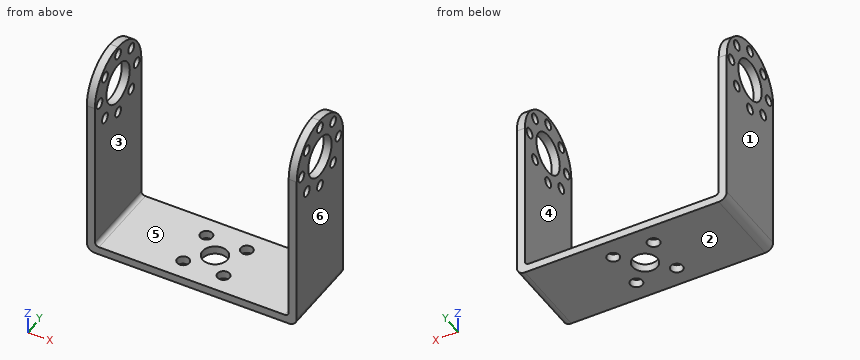
```python
from build123d import *

# Parameters (mm, degrees)
EXTRUDE_1_DEPTH     = 20
FILLET_1_R          = 2
FILLET_2_R          = 1
CUT_EXTRUDE_1_DEPTH = 52
CUT_EXTRUDE_2_DEPTH = 52
SKETCH_4_R          = 5.025
SKETCH_4_R_2        = 1.25
CUT_EXTRUDE_3_DEPTH = 52
CUT_EXTRUDE_4_REACH = 52
SKETCH_5_R          = 3.05
SKETCH_5_R_2        = 1.5


with BuildPart() as part:
    # 草图1 → 凸台-拉伸1 (new body)
    with BuildSketch(Plane(origin=(0, 0, 0), x_dir=(1, 0, 0), z_dir=(0, 1, 0))):
        Polygon((-19.308800698, 32.095662915), (32.691199302, 32.095662915), (32.691199302, -17.904337085), (30.691199302, -17.904337085), (30.691199302, 30.095662915), (-17.308800698, 30.095662915), (-17.308800698, -17.904337085), (-19.308800698, -17.904337085), align=None)
    extrude(amount=EXTRUDE_1_DEPTH)

    # 圆角1
    fillet_1_edges = [part.edges().sort_by_distance(p)[0] for p in [
        (-19.308800698, 10, -32.095662915),
        (32.691199302, 10, -32.095662915),
    ]]
    fillet(fillet_1_edges, radius=FILLET_1_R)

    # 圆角2
    fillet_2_edges = [part.edges().sort_by_distance(p)[0] for p in [
        (30.691199302, 10, -30.095662915),
        (-17.308800698, 10, -30.095662915),
    ]]
    fillet(fillet_2_edges, radius=FILLET_2_R)

    # 草图2 → 切除-拉伸1 (cut)
    with BuildSketch(Plane.ZY.offset(19.308800698)):
        with BuildLine():
            Line((7.904337085, 20), (17.904337085, 20))
            Line((17.904337085, 20), (17.904337085, 10))
            ThreePointArc((17.904337085, 10), (14.975404897, 17.071067812), (7.904337085, 20))
        make_face()
    extrude(amount=-CUT_EXTRUDE_1_DEPTH, mode=Mode.SUBTRACT)

    # 草图3 → 切除-拉伸2 (cut)
    with BuildSketch(Plane.ZY.offset(19.308800698)):
        with BuildLine():
            Line((7.904337085, 0), (17.904337085, 0))
            Line((17.904337085, 0), (17.904337085, 10))
            ThreePointArc((17.904337085, 10), (14.975404897, 2.928932188), (7.904337085, 0))
        make_face()
    extrude(amount=-CUT_EXTRUDE_2_DEPTH, mode=Mode.SUBTRACT)

    # 草图4 → 切除-拉伸3 (cut)
    with BuildSketch(Plane.ZY.offset(19.308800698)):
        with Locations((7.904337085, 10)):
            Circle(SKETCH_4_R)
        with Locations((7.904337085, 18)):
            Circle(SKETCH_4_R_2)
        with Locations((13.561191335, 15.656854249)):
            Circle(SKETCH_4_R_2)
        with Locations((15.904337085, 10)):
            Circle(SKETCH_4_R_2)
        with Locations((13.561191335, 4.343145751)):
            Circle(SKETCH_4_R_2)
        with Locations((7.904337085, 2)):
            Circle(SKETCH_4_R_2)
        with Locations((2.247482836, 4.343145751)):
            Circle(SKETCH_4_R_2)
        with Locations((-0.095662915, 10)):
            Circle(SKETCH_4_R_2)
        with Locations((2.247482836, 15.656854249)):
            Circle(SKETCH_4_R_2)
    extrude(amount=-CUT_EXTRUDE_3_DEPTH, mode=Mode.SUBTRACT)

    # 草图5 → 切除-拉伸4 (cut, up to next)
    with BuildSketch(Plane(origin=(0, 0, -32.095662915), x_dir=(-1, 0, 0), z_dir=(0, 0, -1)), mode=Mode.PRIVATE) as cut_extrude_4_sk1:
        with Locations((-6.691199302, 10)):
            Circle(SKETCH_5_R)
    cut_extrude_4_tool1 = extrude(cut_extrude_4_sk1.sketch, amount=-CUT_EXTRUDE_4_REACH, mode=Mode.PRIVATE) & part.part
    add(cut_extrude_4_tool1.solids().sort_by_distance((6.691199, 10, -32.095663))[0], mode=Mode.SUBTRACT)
    # 草图5 → 切除-拉伸4 (cut, up to next)
    with BuildSketch(Plane(origin=(0, 0, -32.095662915), x_dir=(-1, 0, 0), z_dir=(0, 0, -1)), mode=Mode.PRIVATE) as cut_extrude_4_sk2:
        with Locations((-11.691199302, 15)):
            Circle(SKETCH_5_R_2)
    cut_extrude_4_tool2 = extrude(cut_extrude_4_sk2.sketch, amount=-CUT_EXTRUDE_4_REACH, mode=Mode.PRIVATE) & part.part
    add(cut_extrude_4_tool2.solids().sort_by_distance((11.691199, 15, -32.095663))[0], mode=Mode.SUBTRACT)
    # 草图5 → 切除-拉伸4 (cut, up to next)
    with BuildSketch(Plane(origin=(0, 0, -32.095662915), x_dir=(-1, 0, 0), z_dir=(0, 0, -1)), mode=Mode.PRIVATE) as cut_extrude_4_sk3:
        with Locations((-1.691199302, 15)):
            Circle(SKETCH_5_R_2)
    cut_extrude_4_tool3 = extrude(cut_extrude_4_sk3.sketch, amount=-CUT_EXTRUDE_4_REACH, mode=Mode.PRIVATE) & part.part
    add(cut_extrude_4_tool3.solids().sort_by_distance((1.691199, 15, -32.095663))[0], mode=Mode.SUBTRACT)
    # 草图5 → 切除-拉伸4 (cut, up to next)
    with BuildSketch(Plane(origin=(0, 0, -32.095662915), x_dir=(-1, 0, 0), z_dir=(0, 0, -1)), mode=Mode.PRIVATE) as cut_extrude_4_sk4:
        with Locations((-1.691199302, 5)):
            Circle(SKETCH_5_R_2)
    cut_extrude_4_tool4 = extrude(cut_extrude_4_sk4.sketch, amount=-CUT_EXTRUDE_4_REACH, mode=Mode.PRIVATE) & part.part
    add(cut_extrude_4_tool4.solids().sort_by_distance((1.691199, 5, -32.095663))[0], mode=Mode.SUBTRACT)
    # 草图5 → 切除-拉伸4 (cut, up to next)
    with BuildSketch(Plane(origin=(0, 0, -32.095662915), x_dir=(-1, 0, 0), z_dir=(0, 0, -1)), mode=Mode.PRIVATE) as cut_extrude_4_sk5:
        with Locations((-11.691199302, 5)):
            Circle(SKETCH_5_R_2)
    cut_extrude_4_tool5 = extrude(cut_extrude_4_sk5.sketch, amount=-CUT_EXTRUDE_4_REACH, mode=Mode.PRIVATE) & part.part
    add(cut_extrude_4_tool5.solids().sort_by_distance((11.691199, 5, -32.095663))[0], mode=Mode.SUBTRACT)


solid = part.part
```
Verification items for the finished model (mm, model axes). Face numbers are marked on the shaded views. A direction names the side the tool comes from. Give positions to 0.01 mm unless a question says otherwise; leave off trailing zeros. Order: outer loops, then holes, each group sorted by start corner. A loop starts at its lowest first (then second) coordinate and runs counter-clockwise, first axis right, second up. Notation, with made-up numbers: (-15, -19.5) -> (13, -19.5) arc R27 cw to (13, 5.5) -> close; hole circle Ø6 at (-4, 46). An arc over 180 degrees is marked (long way). Use a Markdown table: item, result.
1) Section check C-C, the plane y = 18. Record the boundary of the cut face in (x, z), then the cut area to 3 significant figures.
Results:
| item | result |
|---|---|
| outline | (-19.31, -30.1) arc R2 ccw to (-17.31, -32.1) -> (30.69, -32.1) arc R2 ccw to (32.69, -30.1) -> (32.69, 6.65) -> (30.69, 6.65) -> (30.69, -29.1) arc R1 cw to (29.69, -30.1) -> (-16.31, -30.1) arc R1 cw to (-17.31, -29.1) -> (-17.31, 6.65) -> (-19.31, 6.65) -> close; (-19.31, 9.15) -> (-17.31, 9.15) -> (-17.31, 13.9) -> (-19.31, 13.9) -> close; (30.69, 9.15) -> (32.69, 9.15) -> (32.69, 13.9) -> (30.69, 13.9) -> close |
| area | 269 mm² |
2) Material ranges on probe 1 along X at (y, z) = (14.75, -28); probe 2 along Z at (x, y) = (-2, 16); probe 3 along Z at (x, y) = (31.5, 9.5), recorded low to high.
Results:
| item | result |
|---|---|
| probe 1 | -19.31 to -17.31, 30.69 to 32.69 |
| probe 2 | -32.1 to -30.1 |
| probe 3 | -31.92 to -1.24, 1.05 to 2.9, 12.9 to 14.76, 17.05 to 17.89 |
3) Section check A-A, the plane z = -18. Record the boundary of the cut face in (x, y).
Results:
| item | result |
|---|---|
| outline | (-19.31, 0) -> (-17.31, 0) -> (-17.31, 20) -> (-19.31, 20) -> close; (30.69, 0) -> (32.69, 0) -> (32.69, 20) -> (30.69, 20) -> close |
4) Mould release check, pull along X, two halves, no side actions. Record for the marked faces 1, 2, 3 and 4: pulls with the +X half, pulls with the -X half, needs draft (parallel to the pull), parting line crosses it, or undercut.
Results:
| item | result |
|---|---|
| face 1 | pulls with the -X half |
| face 2 | needs draft |
| face 3 | undercut |
| face 4 | undercut |
5) Depth check by flat-ended pin: pin 1 Ø5 at (x, y) = (11.69, 15) entering from +Z; pin 2 Ø3 at (y, z) = (10, 15.9) entering from -X; pin 3 Ø2 at (y, z) = (2, 7.9) entering from -X. Enter the tip coordinate at first touch or a pass-through.
Results:
| item | result |
|---|---|
| pin 1 | z = -30.1 |
| pin 2 | x = -19.31 |
| pin 3 | through |
6) Section check D-D, the plane x = -15. Record the boundary of the cut face in (y, z).
Results:
| item | result |
|---|---|
| outline | (0, -32.1) -> (20, -32.1) -> (20, -30.1) -> (0, -30.1) -> close |
7) Section check B-B, the plane x = 5. Record the boundary of the cut face in (y, z).
Results:
| item | result |
|---|---|
| outline | (0, -32.1) -> (7.46, -32.1) -> (7.46, -30.1) -> (0, -30.1) -> close; (12.54, -32.1) -> (20, -32.1) -> (20, -30.1) -> (12.54, -30.1) -> close |
8) Tool access check on the marked faces 5 and 6. Record the directions out of +Z, -Z, +X, -X, +Y, -Y that give a thin tool (end or side, any length) a straight path to the whole face; none if there is none.
Results:
| item | result |
|---|---|
| face 5 | +Z, +Y, -Y |
| face 6 | +Z, -Z, +X, +Y, -Y |
